Autodesk Inventor part; units mm, degrees
ref_plane "Work Plane2" through (5, 3, 2) normal (0, 1, 0) x (1, 0, 0)
ref_plane "Work Plane1" through (0, -3, 18) normal (1, 0, 0) x (0, 0, -1)
ref_plane "YZ Plane" through (0, 0, 0) normal (1, 0, 0) x (0, 1, 0)
sketch "Sketch6" plane through (0, 0, 0) normal (0, 0, 1) x (1, 0, 0)
  line L0 (-5, 5) -> (5, 5)
  line L1 (5, 5) -> (5, -5)
  line L2 (5, -5) -> (-5, -5)
  line L3 (-5, -5) -> (-5, 5)
  point P0 (0, 0)
  dimension "d31" = 10
  dimension "d32" = 10
  dimension "d33" = 5
  dimension "d34" = 5
extrude "Extrusion3" add sketch "Sketch6" along normal blind 20
sketch "Sketch7" plane through (0, 0, 20) normal (0, 0, 1) x (1, 0, 0)
  point P0 (0, 0)
  point P1 (0, 0)
hole "Hole4" at (0, 0, 20) direction (0, 0, -1) diameter 3.1 depth 8
sketch "Sketch8" plane through (-5, 5, 0) normal (0, 1, 0) x (1, 0, 0)
  point P0 (5, 0)
  point P1 (5, -5)
  dimension "d44" = 5
hole "Hole5" at (0, 5, 5) direction (0, -1, 0) diameter 3.3 end through all counterbore diameter 4.1 counterbore depth 5
sketch "Sketch9" plane through (5, -5, 0) normal (1, 0, 0) x (0, 0, -1)
  line L0 (0, 10) -> (-20, 10) construction
  line L1 (-10, 10) -> (-10, 0) construction
  line L2 (0, 0) -> (-20, 0) construction
  line L3 (0, 0) -> (0, 10)
  line L4 (-10, 8) -> (0, 8)
  line L5 (0, 8) -> (0, 2)
  line L6 (0, 2) -> (-10, 2)
  line L7 (-10, 2) -> (-10, 8)
  line L8 (0, 5) -> (-20, 5)
  line L9 (-20, 10) -> (-20, 0)
  dimension "d52" = 6
extrude "Extrusion4" add sketch "Sketch9" along normal blind 15
ref_plane "Work Plane2" through (5, 3, 2) normal (0, 1, 0) x (1, 0, 0)
ref_plane "Work Plane1" through (0, -3, 18) normal (1, 0, 0) x (0, 0, -1)
mirror "Mirror1" about plane through (0, -3, 18) normal (1, 0, 0) of "Extrusion4"
fillet "Fillet3" radius 2 6 edges at (-12.5, 3, 0) (-12.5, 3, 10) (12.5, 3, 10) (-12.5, -3, 10) (12.5, -3, 10) (-12.5, -3, 0)
fillet "Fillet4" radius 2 10 edges at (12.5, 3, 0) (12.5, -3, 0) (5, 5, 10) (-5, 5, 10) (-5, -5, 10) (5, -5, 10) (-5, 0, 20) (5, 0, 20) (0, 5, 20) (0, -5, 20)
fillet "Fillet5" radius 2 14 edges at (20, -2.4144, 0.5856) (20, -3, 4.9997) (20, 0, 0) (20, 2.4144, 0.5856) (20, 3, 4.9997) (20, 0, 10) (-20, 0, 10) (-20, -2.4142, 9.4142) (-20, -3, 5) (-20, -2.4142, 0.5858) (-20, 0, 0) (-20, 2.4142, 0.5858) (-20, 3, 5) (-20, 2.4142, 9.4142)
sketch "Sketch11" plane through (-3, -5, 0) normal (0, -1, 0) x (1, 0, 0)
  circle A0 centre (3, 5) radius 1.65
  point P0 (3, 0)
sketch "Sketch12" plane through (5, 3, 8) normal (0, 1, 0) x (1, 0, 0)
  line L0 (0, 6) -> (0, 0) construction
  line L1 (0, 3) -> (15, 3) construction
  line L2 (15, 0) -> (15, 6) construction
  line L3 (-10, 0) -> (-10, 6) construction
  line L4 (-10, 3) -> (-25, 3) construction
  line L5 (-25, 6) -> (-25, 0) construction
  point P0 (-5, 8)
  point P1 (10, 3)
  point P2 (-20, 3)
  dimension "d67" = 5
  dimension "d68" = 5
hole "Hole7" at (15, 3, 5) at (-15, 3, 5) direction (0, -1, 0) diameter 3.3 end through all counterbore diameter 4.1 counterbore depth 4
CAD build for the part. Positions are in the model's coordinates, mm. A direction names the side the tool comes from. Coordinates: 2 decimals unless noted, no trailing zeros. Write each loop counter-clockwise with the first axis right and the second up, starting at its lowest first coordinate (ties: lowest second). Pieces come first, ordered by that corner, then holes. Notation, with made-up numbers: M 37,-3 L 75,-3 A10 ccw 75,5 Z; hole C 11.5,-27.5 d9. An arc over 180 degrees is marked long. Return JSON: item names as keys, results as strings.
Item 1: Slice it at B-B, the plane z = 17.5. Write the cut outline in (x, y), and give its area (3 significant figures).
Findings below:
{"outline": "M -5,-3 A2 ccw -3,-5 L 3,-5 A2 ccw 5,-3 L 5,3 A2 ccw 3,5 L -3,5 A2 ccw -5,3 Z; hole C 0,0 d3.1", "area": "89.0 mm2"}
Item 2: Slice it at A-A, the plane x = -15. Write the cut outline in (y, z).
Findings below:
{"outline": "M -3,2 A2 ccw -1,0 L 1,0 A2 ccw 3,2 L 3,2.95 L -1,2.95 L -1,3.35 L -3,3.35 Z; M -3,6.65 L -1,6.65 L -1,7.05 L 3,7.05 L 3,8 A2 ccw 1,10 L -1,10 A2 ccw -3,8 Z"}
Item 3: Probe line 1 (X direction, y = 0.9, z = 5); line 2 (Z direction, x = 15, y = 0.85); line 3 (X direction, y = -0.25, z = 3.25). List the from-to ranges inside material, lowest first. Write a range as from..to.
Findings below:
{"line 1": "x = -20..-17.05, -12.95..-2.05, 2.05..12.95, 17.05..20", "line 2": "z = 0..2.95, 7.05..10", "line 3": "x = -20..-16.07, -13.93..13.93, 16.07..20"}
Item 4: Which spindle directions (+Z, -Z, +X, -X, +Y, -Y) get a long thin tool onto all of the face, cutting with end or side? Do faces 1 (the flat face through (-11, 3, 5)), 2 (the cylindrical face through (16.247, 0.972, 3.373)), 3 (the cylindrical face through (-11.59, 2.43, 0.6)), 4 (the flat face through (11, -3, 5)). Say none if no direction does.
Findings below:
{"face 1": "+Z, -Z, -X, +Y", "face 2": "+Y", "face 3": "-Z, -X, +Y", "face 4": "+Z, -Z, +X, -Y"}
Item 5: Drop flat-ended pins along their axis: pin 1 Ø6.5 at (x, z) = (12, 4) entering from -Y; pin 2 Ø5 at (x, z) = (9.5, 6) entering from +Y; pin 3 Ø2 at (y, z) = (4, 12) entering from -X. Give the stop position or say it passes through.
Findings below:
{"pin 1": "stops at y = -3", "pin 2": "stops at y = 3", "pin 3": "stops at x = -5"}
Item 6: Slice it at D-D, the plane x = -10.5. Write the cut outline in (y, z), and give its area (3 significant figures).
Findings below:
{"outline": "M -3,2 A2 ccw -1,0 L 1,0 A2 ccw 3,2 L 3,8 A2 ccw 1,10 L -1,10 A2 ccw -3,8 Z", "area": "56.6 mm2"}
Item 7: Two-plate mould, pull along Z, no slides. Class faces 5 (the cylindrical face through (19.4, -0.01, 0.57)), 6 (the flat face through (11, 0, 10)), 7 (the cylindrical face through (-0.09, 2.46, 2.95)), 8 (the cylindrical face through (19.4, -2.43, 5.04)): +Z half, -Z half, draft (parallel to the pull), parting line (faces both ways), or undercut.
Findings below:
{"face 5": "-Z half", "face 6": "+Z half", "face 7": "undercut", "face 8": "draft"}
Item 8: Slice it at C-C, the plane y = -4.5. Write the cut outline in (x, z), and give its area (3 significant figures).
Findings below:
{"outline": "M -4.32,0 L 4.32,0 L 4.32,18 A1.32 ccw 3,19.32 L -3,19.32 A1.32 ccw -4.32,18 Z; hole C 0,5 d3.3", "area": "158 mm2"}
